The listing builds one solid part. Answer for the finished solid, in the listing's coordinates (mm). Coordinates: 2 decimals unless noted, no trailing zeros. Loops run counter-clockwise (first coordinate to the right, second up) from the corner with the lowest first, then second, coordinate; pieces in that order, holes last. Notation, with made-up numbers: (69.5, -21) - (75.5, -21) arc R29 cw to (75.5, 5) - close; hole circle Ø5 at (57, -1.5). An arc over 180 degrees is marked (long way). Put each result on its own line as item: value.
```python
from build123d import *

# Parameters (mm, degrees)
SKETCH075_W             = 101.6
SKETCH075_H             = 147
PAD026_DEPTH            = 25.4
SKETCH076_W             = 45.794352
SKETCH076_H             = 8.488647
POCKET024_DEPTH         = 5
SKETCH077_R             = 2
POCKET025_DEPTH         = 101.601
BODY015_PLACEMENT_ANGLE = 90


with BuildPart() as part:
    # Sketch075 → Pad026 (new body)
    with BuildSketch(Plane.XY):
        Rectangle(SKETCH075_W, SKETCH075_H)
    extrude(amount=PAD026_DEPTH)

    # Sketch076 (on Face3 of Pad026) → Pocket024 (cut)
    with BuildSketch(Plane(origin=(0, 73.5, 0), x_dir=(-1, 0, 0), z_dir=(0, 1, 0))):
        with Locations((-19.708751, 4.2443235)):
            Rectangle(SKETCH076_W, SKETCH076_H)
    extrude(amount=-POCKET024_DEPTH, mode=Mode.SUBTRACT)

    # Sketch077 (on Face2 of Pocket024) → Pocket025 (cut, through all)
    with BuildSketch(Plane(origin=(-50.8, 0, 0), x_dir=(0, -1, 0), z_dir=(-1, 0, 0))):
        with Locations((-45, 6.35)):
            Circle(SKETCH077_R)
        with Locations((56.6, 6.35)):
            Circle(SKETCH077_R)
    extrude(amount=-POCKET025_DEPTH, mode=Mode.SUBTRACT)


with BuildPart() as part_1:
    # Body015 placement: moved
    add(part.part.moved(Location((281.1, 101.86, 14.7))).rotate(Axis((281.1, 101.86, 14.7), (0, 0, 1)), BODY015_PLACEMENT_ANGLE))


solid = part_1.part
```
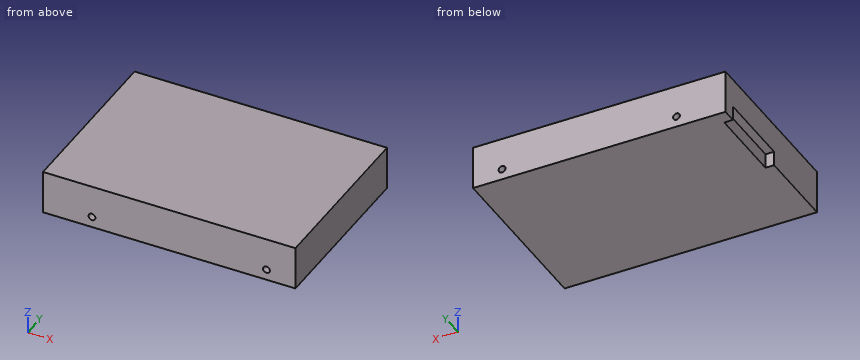
1) Each of these flat-tipped pins is pushed along its axis until it touches: pin 1 (4 mm diameter, centred on y = 121.5, z = 17, fed in from -X); pin 2 (1.5 mm diameter, centred on x = 210, y = 131.5, fed in from -Z). Where does it stop, or does it pass through?
Found:
pin 1: stops at x = 212.6
pin 2: stops at z = 23.19
2) The part is cut by section C-C (z = 21.05). Give the vertices of the cut face in (x, y), and give its area (3 significant figures).
Found:
outline: (207.6, 51.06) - (234.1, 51.06) - (234.1, 152.66) - (207.6, 152.66) - (207.6, 144.47) - (212.6, 144.47) - (212.6, 98.67) - (207.6, 98.67) - close; (238.1, 51.06) - (335.7, 51.06) - (335.7, 152.66) - (238.1, 152.66) - close; (339.7, 51.06) - (354.6, 51.06) - (354.6, 152.66) - (339.7, 152.66) - close
area: 13,900 mm^2
3) Straight lines are drawn through the part: L1, parallel to Z at x = 236, y = 111; L2, parallel to X at y = 65, z = 21.5; L3, parallel to X at y = 134, z = 22. For each, find the intervals that lie inside material, in ascending order. Write a range as [from, to].
Found:
L1: z = [14.7, 19.05], [23.05, 40.1]
L2: x = [207.6, 234.15], [238.05, 335.75], [339.65, 354.6]
L3: x = [212.6, 234.34], [237.86, 335.94], [339.46, 354.6]
4) The part is cut by section A-A (y = 112). Give the vertices of the cut face in (x, z).
Found:
outline: (207.6, 23.19) - (212.6, 23.19) - (212.6, 14.7) - (354.6, 14.7) - (354.6, 40.1) - (207.6, 40.1) - close; hole circle Ø4 at (236.1, 21.05); hole circle Ø4 at (337.7, 21.05)
5) The part is cut by section B-B (x = 236.1). Give the vertices of the cut face in (y, z).
Found:
outline: (51.06, 14.7) - (152.66, 14.7) - (152.66, 19.05) - (51.06, 19.05) - close; (51.06, 23.05) - (152.66, 23.05) - (152.66, 40.1) - (51.06, 40.1) - close
